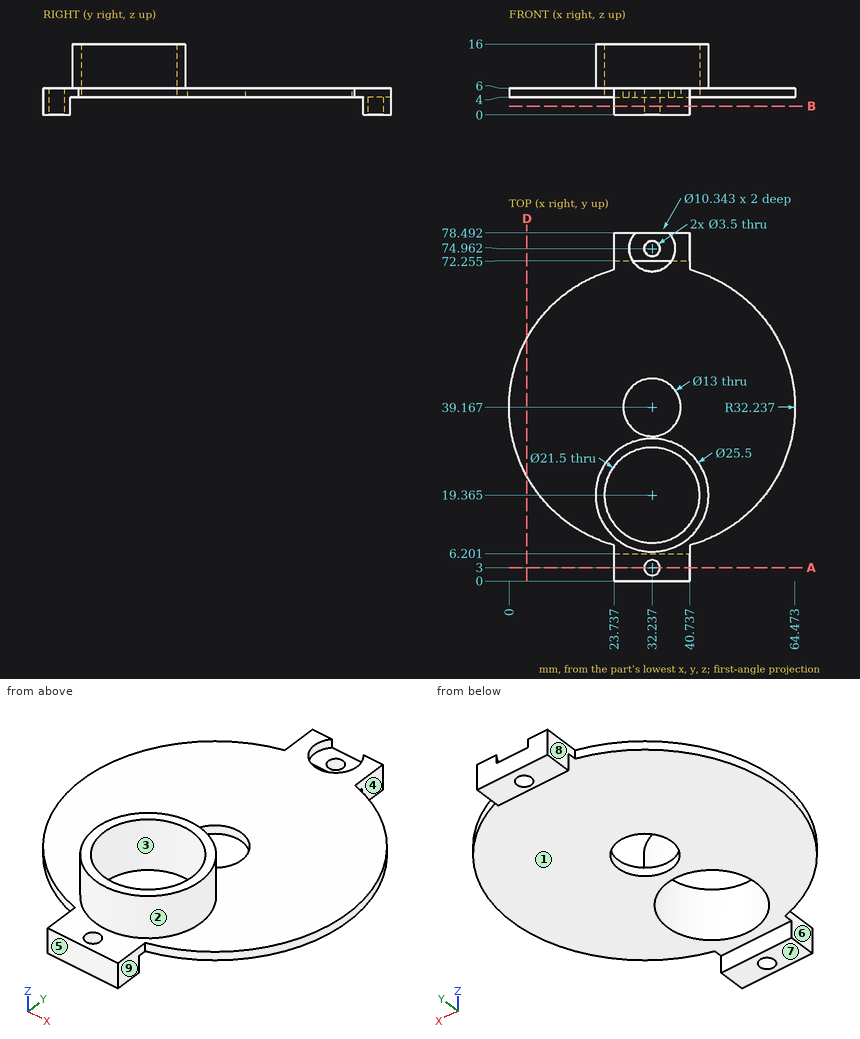
Study the drawing (mm; zero at the part's minimum x, y, z) and answer. A direction names the side the tool comes from. Coordinates: 2 decimals unless noted, no trailing zeros. Order: outer loops, then holes, each group sorted by start corner. A loop starts at its lowest first (then second) coordinate and runs counter-clockwise, first axis right, second up. Notation, with made-up numbers: M 14.25,-15 L 72.25,-15 A26 cw 72.25,10 Z; hole C 34.25,82.5 d8. An arc over 180 degrees is marked long. Use CSV: the item, a comma, the result in double quotes.
Q1. Section A-A (y = 3) is taken. Determine the outline of the cut face in (x, z).
Here are the results:
outline,"M 23.74,0 L 30.49,0 L 30.49,6 L 23.74,6 Z; M 33.99,0 L 40.74,0 L 40.74,6 L 33.99,6 Z"
Q2. Straight lines are drawn through the part: L1, parallel to X at y = 3, z = 2.2; L2, parallel to Z at x = 46, y = 59; L3, parallel to Y at x = 41, z = 13.75 (1 decimal). For each, find the intervals that lie inside material, in ascending order.
Here are the results:
L1,"23.74 to 30.49, 33.99 to 40.74"
L2,"4 to 6"
L3,"10.1 to 13.1, 25.6 to 28.6"
Q3. A tool of negligible diameter and unlimited length cuts with its end or side. For the marked faces 5, 6, 7, 8 and 9, from which of +Z, -Z, +X, -X, +Y, -Y can it reach the whole face along a straight path? Write none if from no direction.
Here are the results:
face 5,"+Z, -Z, +X, -X, -Y"
face 6,"+Z, -Z, -X, -Y"
face 7,"-Z, +X, -X, +Y, -Y"
face 8,"+Z, -Z, -X, +Y"
face 9,"+Z, -Z, +X, -Y"
Q4. Section B-B (z = 2) is taken. Give the number of separate pieces and of enclosed holes in the cut face, then the cut area to 3 significant figures.
Here are the results:
separate pieces,"2"
enclosed holes,"2"
area,"192 mm2"
Q5. Determine the mould class of the marked faces 1, 2, 3 and 4 for opening direction Y: pulls with the +Y half, pulls with the -Y half, needs draft (parallel to the pull), parting line crosses it, or undercut.
Here are the results:
face 1,"undercut"
face 2,"parting line crosses it"
face 3,"undercut"
face 4,"needs draft"
Q6. Section D-D (x = 4) is taken. Determine the outline of the cut face in (y, z) (1 decimal).
Here are the results:
outline,"M 23.6,4 L 54.7,4 L 54.7,6 L 23.6,6 Z"
Q7. Given pin 1 Ø3 at (y, z) = (4, 2.5) entering from +X; pin 2 Ø16.5 at (x, y) = (32.24, 74.96) entering from +Z; pin 3 Ø5 at (y, z) = (2.5, 4.5) entering from -X, each flat-ended and moving along its own axis, determine where each tip first touches the part or whether it passes through.
Here are the results:
pin 1,"x = 40.74"
pin 2,"z = 6"
pin 3,"x = 23.74"
